Read the model definition and answer for the solid it produces. Units are mm, in the model's axes. A direction names the side the tool comes from. Round coordinates to 2 decimals unless told otherwise and drop trailing zeros. Order: outer loops, then holes, each group sorted by start corner. A loop starts at its lowest first (then second) coordinate and runs counter-clockwise, first axis right, second up. Notation, with made-up numbers: (-5.75, -2.75) - (35.25, -2.75) arc R20 cw to (35.25, 29.25) - close; hole circle Ø10 at (-14.5, -15.5). An arc over 180 degrees is marked (long way). Answer as a JSON object with one key per item and string values. Group by question number.
Q1. A cutting plane is placed at B-B on z = -4. Determine the outline of the cut face in (x, y), and give its area (3 significant figures).
Q2. A tool of negligible diameter and unlimited length cuts with its end or side. For faces 4 (the flat face through (12.5, 322, 0)), 5 (the cylindrical face through (-5.554, 157.76, 13.394)), 6 (the flat face through (-1, 323, 0)), from which of +Z, -Z, +X, -X, +Y, -Y can it reach the whole face along a straight path? Write none if from no direction.
Q3. Given pin 1 Ø12 at (y, z) = (43, 10) entering from -X; pin 2 Ø3 at (x, z) = (3, 3.5) entering from -Y; pin 3 Ø8.5 at (x, z) = (-7.5, 3) entering from +Y; pin 4 Ø5 at (x, y) = (-12, 325) entering from +Z, each flat-ended and moving along its own axis, determine where each tip first touches the part or whether it passes through.
Q4. A cutting plane is placed at C-C on y = 256. Determine the outline of the cut face in (x, z), and give its area (3 significant figures).
Q5. The mould has two halves that part along X. Classify faces 1 (the flat face through (0, 320, 0)), 2 (the flat face through (-15.5, 322, 0)), 3 (the flat face through (-1, 325, 14.5)): pulls with the +X half, pulls with the -X half, needs draft (parallel to the pull), parting line crosses it, or undercut.
Q6. Consider line 1 (X direction, y = 325, z = -15); line 2 (Y direction, x = -12, z = -16.7); line 3 (Z direction, x = 4, y = 290). Determine where each line is inside the solid, lowest interval first.
Q7. A cutting plane is placed at A-A on x = 0. Determine the outline of the cut face in (y, z), and give its area (4 significant figures).
```python
from build123d import *

# Parameters (mm, degrees)
SKETCH1_R           = 14.5
BOSS_EXTRUDE1_DEPTH = 320
SHELL1_T            = -3
SKETCH2_W           = 28
SKETCH2_H           = 8
BOSS_EXTRUDE2_DEPTH = 17.5
SKETCH4_W           = 29
SKETCH4_H           = 5
CUT_EXTRUDE1_DEPTH  = 28
CUT_EXTRUDE2_REACH  = 332.226
SKETCH5_R           = 1.5


with BuildPart() as part:
    # Sketch1 → Boss-Extrude1 (new body)
    with BuildSketch(Plane(origin=(0, 0, 0), x_dir=(1, 0, 0), z_dir=(0, 1, 0))):
        with Locations(Location((0, 0, 0), (0, 0, 270))):
            Circle(SKETCH1_R)
    extrude(amount=BOSS_EXTRUDE1_DEPTH)

    # Shell1
    shell1_openings = [part.faces().sort_by_distance(p)[0] for p in [
        (0, 320, 0),
        (0, 0, 0),
    ]]
    offset(amount=SHELL1_T, openings=shell1_openings, kind=Kind.INTERSECTION)

    # Sketch2 → Boss-Extrude2 (add, symmetric)
    with BuildSketch(Plane.XY):
        with Locations((-1.5, 324)):
            Rectangle(SKETCH2_W, SKETCH2_H)
    extrude(amount=BOSS_EXTRUDE2_DEPTH, both=True)

    # Sketch4 → Cut-Extrude1 (cut)
    with BuildSketch(Plane(origin=(12.5, 0, 0), x_dir=(0, 0, -1), z_dir=(1, 0, 0))):
        with Locations((0, 325.5)):
            Rectangle(SKETCH4_W, SKETCH4_H)
    extrude(amount=-CUT_EXTRUDE1_DEPTH, mode=Mode.SUBTRACT)

    # Cut-Extrude2: up to this face of the body (flat: up to its plane)
    cut_extrude2_end = Plane(part.part.faces().sort_by_distance((-1.5, 324, -17.5))[0])
    # Sketch5 → Cut-Extrude2 (cut, up to the picked face)
    with BuildSketch(Plane.XY.offset(17.5), mode=Mode.PRIVATE) as cut_extrude2_sk1:
        with Locations((-8, 325)):
            Circle(SKETCH5_R)
    cut_extrude2_tool1 = split(extrude(cut_extrude2_sk1.sketch, amount=-CUT_EXTRUDE2_REACH, mode=Mode.PRIVATE), bisect_by=cut_extrude2_end, keep=Keep.BOTH, mode=Mode.PRIVATE)
    # Sketch5 → Cut-Extrude2 (cut, up to the picked face)
    with BuildSketch(Plane.XY.offset(17.5), mode=Mode.PRIVATE) as cut_extrude2_sk2:
        with Locations((5, 325)):
            Circle(SKETCH5_R)
    cut_extrude2_tool2 = split(extrude(cut_extrude2_sk2.sketch, amount=-CUT_EXTRUDE2_REACH, mode=Mode.PRIVATE), bisect_by=cut_extrude2_end, keep=Keep.BOTH, mode=Mode.PRIVATE)
    # Sketch5 → Cut-Extrude2 (cut, up to the picked face)
    with BuildSketch(Plane.XY.offset(17.5), mode=Mode.PRIVATE) as cut_extrude2_sk3:
        with Locations((9, 325)):
            Circle(SKETCH5_R)
    cut_extrude2_tool3 = split(extrude(cut_extrude2_sk3.sketch, amount=-CUT_EXTRUDE2_REACH, mode=Mode.PRIVATE), bisect_by=cut_extrude2_end, keep=Keep.BOTH, mode=Mode.PRIVATE)
    # Sketch5 → Cut-Extrude2 (cut, up to the picked face)
    with BuildSketch(Plane.XY.offset(17.5), mode=Mode.PRIVATE) as cut_extrude2_sk4:
        with Locations((-12, 325)):
            Circle(SKETCH5_R)
    cut_extrude2_tool4 = split(extrude(cut_extrude2_sk4.sketch, amount=-CUT_EXTRUDE2_REACH, mode=Mode.PRIVATE), bisect_by=cut_extrude2_end, keep=Keep.BOTH, mode=Mode.PRIVATE)
    add(cut_extrude2_tool1.solids().sort_by(Axis((-8, 325, 17.5), (0, 0, -1)))[0], mode=Mode.SUBTRACT)
    add(cut_extrude2_tool2.solids().sort_by(Axis((5, 325, 17.5), (0, 0, -1)))[0], mode=Mode.SUBTRACT)
    add(cut_extrude2_tool3.solids().sort_by(Axis((9, 325, 17.5), (0, 0, -1)))[0], mode=Mode.SUBTRACT)
    add(cut_extrude2_tool4.solids().sort_by(Axis((-12, 325, 17.5), (0, 0, -1)))[0], mode=Mode.SUBTRACT)


solid = part.part
```
Result set:
{
 "1": {"outline": "(-15.5, 320) - (-13.94, 320) - (-13.94, 0) - (-10.78, 0) - (-10.78, 320) - (10.78, 320) - (10.78, 0) - (13.94, 0) - (13.94, 320) - (12.5, 320) - (12.5, 323) - (-15.5, 323) - close", "area": "2,100 mm²"},
 "2": {"face 4": "+Z, -Z, +X, +Y", "face 5": "-Y", "face 6": "+X, -X, +Y"},
 "3": {"pin 1": "stops at x = -13.94", "pin 2": "stops at y = 320", "pin 3": "stops at y = 323", "pin 4": "stops at z = 17.5"},
 "4": {"outline": "circle Ø29 at (0, 0); hole circle Ø23 at (0, 0)", "area": "245 mm²"},
 "5": {"face 1": "undercut", "face 2": "pulls with the -X half", "face 3": "needs draft"},
 "6": {"line 1": "x = -15.5 to -13.5, -10.5 to -9.5, -6.5 to 3.5, 6.5 to 7.5, 10.5 to 12.5", "line 2": "y = 320 to 323.5, 326.5 to 328", "line 3": "z = -13.94 to -10.78, 10.78 to 13.94"},
 "7": {"outline": "(0, -14.5) - (320, -14.5) - (320, -17.5) - (328, -17.5) - (328, -14.5) - (323, -14.5) - (323, 14.5) - (328, 14.5) - (328, 17.5) - (320, 17.5) - (320, 14.5) - (0, 14.5) - (0, 11.5) - (320, 11.5) - (320, -11.5) - (0, -11.5) - close", "area": "2,055 mm²"}
}
